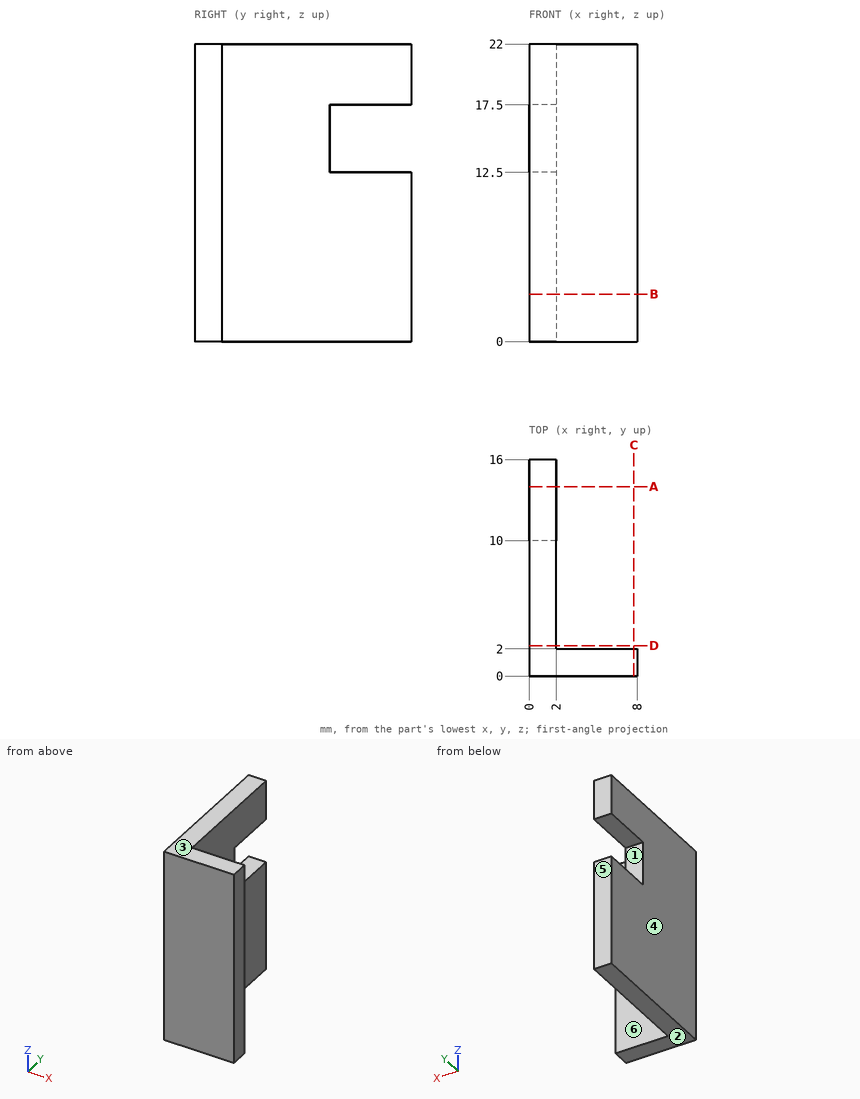
Part print with two shaded views. Sizes in mm from the minimum x, y, z corner. A direction names the side the tool comes from. Give positions to 0.01 mm unless a question says otherwise; leave off trailing zeros. Write each loop counter-clockwise with the first axis right and the second up, starting at its lowest first coordinate (ties: lowest second). Pieces come first, ordered by that corner, then holes.
1) Pin check, flat tips, straight feed: pin 1 (4 mm diameter, centred on x = 6.5, z = 19.5, fed in from +Y); pin 2 (1.6 mm diameter, centred on x = 1, z = 15.5, fed in from +Y). Stop position of each tip, or through.
Resolved:
pin 1: stops at y = 2
pin 2: stops at y = 10
2) Probe L1, parallel to Z at x = 1.75, y = 15; L2, parallel to Y at x = 5, z = 11. List the from-to ranges inside material, lowest first.
Resolved:
L1: z = 0 to 12.5, 17.5 to 22
L2: y = 0 to 2
3) Two-plate mould, pull along Z, no slides. Class the marked faces 1, 2, 3 and 4: released by +Z, released by -Z, zero draft, split by the parting line, or undercut.
Resolved:
face 1: undercut
face 2: released by -Z
face 3: released by +Z
face 4: zero draft
4) Cut at C-C on x = 7.75. Write the cut outline in (y, z).
Resolved:
outline: (0, 0) - (2, 0) - (2, 22) - (0, 22) - close
5) Cut at A-A on y = 14. Write the cut outline in (x, z), then the cut area to 3 significant figures.
Resolved:
outline: (0, 0) - (2, 0) - (2, 12.5) - (0, 12.5) - close; (0, 17.5) - (2, 17.5) - (2, 22) - (0, 22) - close
area: 34.0 mm2
6) Cut at B-B on z = 3.5. Write the cut outline in (x, y).
Resolved:
outline: (0, 0) - (8, 0) - (8, 2) - (2, 2) - (2, 16) - (0, 16) - close
7) Which spindle directions (+Z, -Z, +X, -X, +Y, -Y) get a long thin tool onto all of the face, cutting with end or side? Do the marked faces 5 and 6. Say none if no direction does.
Resolved:
face 5: +Z, -Z, +X, -X, +Y
face 6: +Z, -Z, +X, +Y
